Autodesk Inventor part; units mm, degrees
ref_plane "YZ Plane" through (0, 0, 0) normal (1, 0, 0) x (0, 1, 0)
ref_plane "XZ Plane" through (0, 0, 0) normal (0, 1, 0) x (-1, 0, 0)
ref_plane "XY Plane" through (0, 0, 0) normal (0, 0, 1) x (1, 0, 0)
sketch "Skizze1" plane through (0, 0, 0) normal (0, 0, 1) x (1, 0, 0)
  line L0 (-4.2593, -15) -> (-4.2593, 15) construction
  line L1 (-4.2593, -15) -> (4.6613, -15) construction
  arc A0 (71.1407, -18.3849) -> (4.6613, -15) centre (32.8959, -114.9901) ccw construction
  line L2 (71.1407, -12.6613) -> (71.1407, -18.3849) construction
  line L3 (72.2593, -12.6613) -> (71.1407, -12.6613) construction
  line L4 (72.2593, -19) -> (72.2593, -12.6613) construction
  line L5 (75.2593, -19) -> (72.2593, -19) construction
  line L6 (75.2593, -9.9704) -> (75.2593, -19) construction
  arc A1 (75.2593, -9.9704) -> (13.1677, 13.0021) centre (8.1722, -95.8991) ccw construction
  arc A2 (11.2593, 15) -> (13.1677, 13.0021) centre (13.2593, 15) ccw construction
  line L7 (11.2593, 15) -> (-4.2593, 15) construction
  arc A3 (7.8907, 11.0161) -> (3.5907, 11.0161) centre (5.7407, 11.0161) ccw construction
  line L8 (7.8907, 6.0161) -> (7.8907, 11.0161) construction
  arc A4 (3.5907, 6.0161) -> (7.8907, 6.0161) centre (5.7407, 6.0161) ccw construction
  line L9 (3.5907, 11.0161) -> (3.5907, 6.0161) construction
  line L10 (7.8907, -10.5786) -> (7.8907, -5.5786) construction
  arc A5 (3.5907, -10.5786) -> (7.8907, -10.5786) centre (5.7407, -10.5786) ccw construction
  line L11 (3.5907, -5.5786) -> (3.5907, -10.5786) construction
  arc A6 (7.8907, -5.5786) -> (3.5907, -5.5786) centre (5.7407, -5.5786) ccw construction
  arc A7 (77.2593, -11.57) -> (68.4849, -5.0872) centre (8.1722, -95.8991) ccw construction
  arc A8 (68.4849, -5.0872) -> (68.1407, -6.2089) centre (70.1407, -6.2089) ccw construction
  line L12 (68.1407, -19.3793) -> (68.1407, -6.2089) construction
  arc A9 (71.1407, -20.5393) -> (68.1407, -19.3793) centre (32.8959, -114.9901) ccw construction
  line L13 (71.1407, -13) -> (71.1407, -20.5393) construction
  line L14 (73.1277, -13) -> (71.1407, -13) construction
  line L15 (73.1277, -21) -> (73.1277, -13) construction
  line L16 (77.2593, -21) -> (73.1277, -21) construction
  line L17 (77.2593, -11.57) -> (77.2593, -21) construction
  arc A10 (67.1407, -2.4739) -> (65.1407, -4.4739) centre (67.1407, -4.4739) ccw construction
  line L18 (67.1407, -2.4739) -> (68.1407, -2.4739) construction
  line L19 (68.1407, -2.4739) -> (68.1407, -14.8476) construction
  line L20 (22.4305, -2.4739) -> (87.7065, -2.4739)
  line L21 (87.7065, -2.4739) -> (87.7065, 11.9632)
  line L22 (87.7065, 11.9632) -> (22.4305, 11.9632)
  line L23 (22.4305, 11.9632) -> (22.4305, -2.4739)
  line L24 (26.0799, -2.4739) -> (26.0799, 7.5261) construction
  line L25 (47.5033, 11.9632) -> (47.5033, 1.9632) construction
  circle A11 centre (26.0799, 7.5261) radius 2.15
  circle A12 centre (47.5033, 1.9632) radius 2.15
  point P0 (0, 0)
  dimension "d0" = 10
  dimension "d1" = 10
  dimension "d2" = 4.3
  dimension "d3" = 4.3
extrude "Extrusion1" add sketch "Skizze1" along normal blind 3
sketch "Skizze2" plane through (0, 0, 0) normal (0, 0, -1) x (-1, 0, 0)
  arc A0 (-72.5805, 2.9132) -> (-72.5805, 6.2132) centre (-72.5805, 4.5632) ccw construction
  arc A1 (-73.5805, 6.2132) -> (-73.5805, 2.9132) centre (-73.5805, 4.5632) ccw construction
  arc A2 (-80.2805, 2.9132) -> (-80.2805, 6.2132) centre (-80.2805, 4.5632) ccw construction
  arc A3 (-81.2805, 6.2132) -> (-81.2805, 2.9132) centre (-81.2805, 4.5632) ccw construction
  circle A4 centre (-73.1179, 4.5632) radius 1.6
  circle A5 centre (-80.7335, 4.5632) radius 1.6
  point P0 (0, 0)
  dimension "d6" = 3.2
  dimension "d7" = 3.2
extrude "Extrusion2" cut sketch "Skizze2" against normal through all
fillet "Rundung1" radius 2 2 edges at (55.0685, 11.9632, 3) (87.7065, 4.7446, 3)
fillet "Rundung2" radius 2 3 edges at (87.1208, -2.4739, 2.4142) (87.7065, -2.4739, 0.5) (54.0685, -2.4739, 3)
properties part number "Chain_drag"
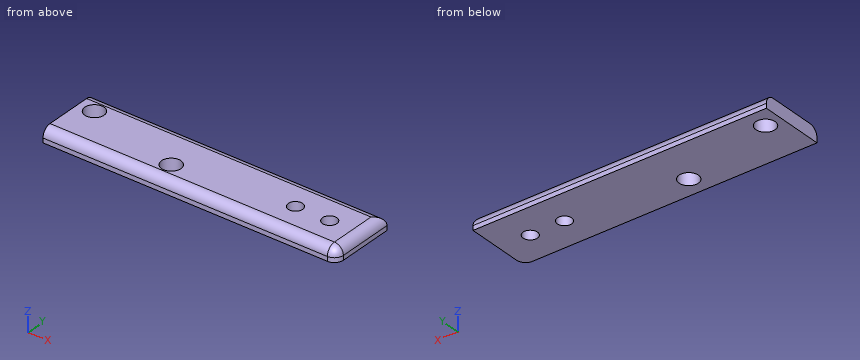
Can you work these out from the model? Positions are in its coordinate system, mm. Round coordinates to 2 decimals unless told otherwise and drop trailing zeros. Loops run counter-clockwise (first coordinate to the right, second up) from the corner with the lowest first, then second, coordinate; pieces in that order, holes last. Notation, with made-up numbers: (-20, -4) - (18, -4) arc R26 cw to (18, 10) - close; hole circle Ø3 at (19.25, 16.5). An arc over 180 degrees is marked (long way). Answer in a Markdown table with one row per item. Add a question column.
Q1. I want a section at B-B on z = 1.45. List the corners of the cut face in (x, y) for me, and give its area (3 significant figures).
Q2. I want a section at A-A on x = 27. List the corners of the cut face in (y, z) for me.
Q3. I want a section at C-C on x = 77. List the corners of the cut face in (y, z) for me, and give its area (3 significant figures).
Q4. For pin 1 Ø3.5 at (x, y) = (80.73, 4.56) entering from +Z, with a flat end and sliding along its axis, tell me the tip position at first contact or that it passes through.
Q5. I need wall thicknesses on L1, parallel to Y at x = 73, z = 1.8; L2, parallel to X at y = 9.5, z = 1.5; L3, parallel to Y at x = 27.5, z = 0.4. Which ranges of each line are inside material? Lowest first, please.
Q6. I want a section at D-D on y = 10.75. List the corners of the cut face in (x, z) for me.
A:
| question | item | result |
|---|---|---|
| 1 | outline | (22.43, -2.42) - (85.71, -2.42) arc R1.95 ccw to (87.66, -0.47) - (87.66, 11.91) - (22.43, 11.91) - close; hole circle Ø4.3 at (26.08, 7.53); hole circle Ø4.3 at (47.5, 1.96); hole circle Ø3.2 at (73.12, 4.56); hole circle Ø3.2 at (80.73, 4.56) |
| 1 | area | 889 mm^2 |
| 2 | outline | (-2.47, 0) - (5.58, 0) - (5.58, 3) - (-0.47, 3) arc R2 ccw to (-2.47, 1) - close; (9.47, 0) - (11.96, 0) - (11.96, 1) arc R2 ccw to (9.96, 3) - (9.47, 3) - close |
| 3 | outline | (-2.47, 0) - (11.96, 0) - (11.96, 1) arc R2 ccw to (9.96, 3) - (-0.47, 3) arc R2 ccw to (-2.47, 1) - close |
| 3 | area | 41.6 mm^2 |
| 4 | pin 1 | z = 3 |
| 5 | L1 | -2.31 to 2.97, 6.16 to 11.8 |
| 5 | L2 | 22.43 to 25.23, 26.93 to 87.64 |
| 5 | L3 | -2.47 to 5.91, 9.14 to 11.96 |
| 6 | outline | (22.43, 0) - (87.71, 0) - (87.71, 1) arc R2 ccw to (86.49, 2.84) - (22.43, 2.84) - close |
